Design review of the part built by this model. Coordinates are the model's own, in mm. A direction names the side the tool comes from. Coordinates: 2 decimals unless noted, no trailing zeros. Order: outer loops, then holes, each group sorted by start corner. A loop starts at its lowest first (then second) coordinate and runs counter-clockwise, first axis right, second up. Notation, with made-up numbers: M 60,10.25 L 69,10.25 A20 cw 69,32.25 Z; hole C 89,18 d9. An arc over 180 degrees is marked long. Answer in a Markdown table with one row per item.
from build123d import *

# Parameters (mm, degrees)
F0_W     = 440
F0_H     = 402
F0_W_2   = 175
F0_H_2   = 156
F1_DEPTH = 10
F2_R     = 20


with BuildPart() as f1:
    # F0 (on Front) → F1 (new body)
    with BuildSketch(Plane.XZ):
        with Locations((-36.484095, -5.070948)):
            Rectangle(F0_W, F0_H)
        with Locations((-138.984095, -98.070948)):
            Rectangle(F0_W_2, F0_H_2, mode=Mode.SUBTRACT)
        with Locations((66.015905, -98.070948)):
            Rectangle(F0_W_2, F0_H_2, mode=Mode.SUBTRACT)
        with Locations((-138.984095, 87.929052)):
            Rectangle(F0_W_2, F0_H_2, mode=Mode.SUBTRACT)
        with Locations((66.015905, 87.929052)):
            Rectangle(F0_W_2, F0_H_2, mode=Mode.SUBTRACT)
    extrude(amount=F1_DEPTH)

    # F2
    f2_edges = [f1.edges().sort_by_distance(p)[0] for p in [
        (153.515905, -5, 165.929052),
        (-21.484095, -5, 165.929052),
        (-226.484095, -5, 165.929052),
        (-226.484095, -5, -20.070948),
        (-21.484095, -5, -20.070948),
        (-51.484095, -5, 165.929052),
        (-51.484095, -5, 9.929052),
        (-51.484095, -5, -176.070948),
        (153.515905, -5, -176.070948),
        (153.515905, -5, 9.929052),
        (-226.484095, -5, -176.070948),
        (-226.484095, -5, 9.929052),
        (-21.484095, -5, -176.070948),
        (-21.484095, -5, 9.929052),
        (-51.484095, -5, -20.070948),
        (153.515905, -5, -20.070948),
    ]]
    fillet(f2_edges, radius=F2_R)


solid = f1.part
(1) Draft analysis for pull direction X (two halves, no side actions). For faces 3 (the cylindrical face through (-220.47, -5.07, -170.37)), 4 (the flat face through (183.516, -5, -8)), 5 (the cylindrical face through (-15.781, -5.07, -26.085)), 6 (the flat face through (-40, -10, -2)), state which applies: pulls with the +X half, pulls with the -X half, needs draft (parallel to the pull), parting line crosses it, or undercut.
Return value:
| item | result |
|---|---|
| face 3 | undercut |
| face 4 | pulls with the +X half |
| face 5 | undercut |
| face 6 | needs draft |
(2) Add section A-A, the plane x = 106. Give the boundary of the cut face in (y, z).
Return value:
| item | result |
|---|---|
| outline | M -10,-206.07 L 0,-206.07 L 0,-176.07 L -10,-176.07 Z; M -10,-20.07 L 0,-20.07 L 0,9.93 L -10,9.93 Z; M -10,165.93 L 0,165.93 L 0,195.93 L -10,195.93 Z |
(3) Add section C-C, the plane y = -1.5. Give the number of separate pieces and of enclosed holes in the cut face, and give its area (3 significant figures).
Return value:
| item | result |
|---|---|
| separate pieces | 1 |
| enclosed holes | 4 |
| area | 69,100 mm2 |
(4) For line 1 along X through (y, z) = (-3.5, 143); line 2 along Z through (x, y) = (123.5, -4.5); line 3 along Z through (x, y) = (-64, -4), list the stretches that pass through material, from the lowest coordinate up. Write a range as from..to.
Return value:
| item | result |
|---|---|
| line 1 | x = -256.48..-226.48, -51.48..-21.48, 153.52..183.52 |
| line 2 | z = -206.07..-176.07, -20.07..9.93, 165.93..195.93 |
| line 3 | z = -206.07..-174.62, -21.52..11.38, 164.48..195.93 |
(5) Add section B-B, the plane z = -119. Give the boundary of the cut face in (x, y), and give its area (3 significant figures).
Return value:
| item | result |
|---|---|
| outline | M -256.48,-10 L -226.48,-10 L -226.48,0 L -256.48,0 Z; M -51.48,-10 L -21.48,-10 L -21.48,0 L -51.48,0 Z; M 153.52,-10 L 183.52,-10 L 183.52,0 L 153.52,0 Z |
| area | 900 mm2 |
(6) For faces 1 (the flat face through (-256.484, -5, -8)), 2 (the flat face through (153.516, -5, 87)), list the 3-axis set-ups (+Z, -Z, +X, -X, +Y, -Y) from which the entire face can be reached by the end or side of a thin tool; tool diameter is ignored.
Return value:
| item | result |
|---|---|
| face 1 | +Z, -Z, -X, +Y, -Y |
| face 2 | +Y, -Y |
